Geometry: final body of the model. Coordinates: model frame, mm. Face numbers are marked on the shaded views. A direction names the side the tool comes from. Give positions to 0.01 mm unless a question says otherwise; leave off trailing zeros. Order: outer loops, then holes, each group sorted by start corner. A loop starts at its lowest first (then second) coordinate and runs counter-clockwise, first axis right, second up. Notation, with made-up numbers: M -17.5,-14 L 31.5,-14 A31 ccw 31.5,13 Z; hole C -32,89.5 d10. An arc over 180 degrees is marked long. One line per item, written item: value. Start each with the question number.
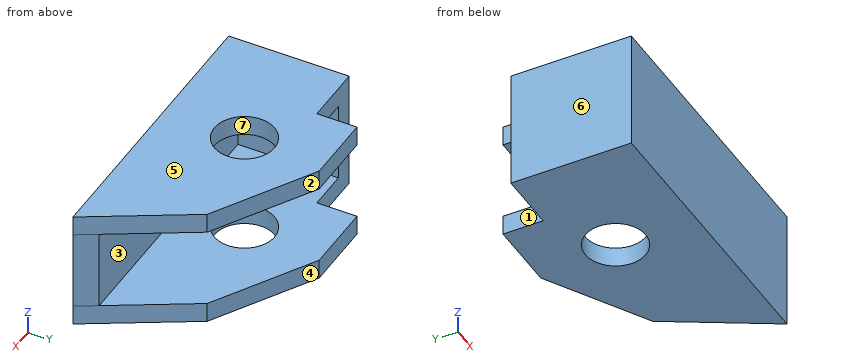
Autodesk Inventor part; units mm, degrees
ref_plane "YZ Plane" through (0, 0, 0) normal (1, 0, 0) x (0, 1, 0)
ref_plane "XZ Plane" through (0, 0, 0) normal (0, 1, 0) x (-1, 0, 0)
ref_plane "XY Plane" through (0, 0, 0) normal (0, 0, 1) x (1, 0, 0)
sketch "Sketch1" plane through (0, 0, 0) normal (0, 0, 1) x (1, 0, 0)
  line L0 (0, 0) -> (91.948, 0)
  line L1 (0, 0) -> (0, 38.1)
  line L2 (0, 38.1) -> (19.05, 38.1)
  line L3 (19.05, 38.1) -> (19.05, 50.8)
  line L4 (19.05, 50.8) -> (41.402, 50.8)
  line L5 (91.948, 0) -> (223.0777, 0) construction
  line L6 (41.402, 50.8) -> (73.2269, 32.4259)
  line L7 (91.948, 0) -> (73.2269, 32.4259)
  circle A0 centre (38.1, 25.4) radius 9.525
  dimension "d3" = 12.7
  dimension "d7" = 19.05
  dimension "d8" = 50.8
  dimension "d9" = 41.402
  dimension "d10" = 60
  dimension "d11" = 30
  dimension "d12" = 19.05
  dimension "d13" = 38.1
  dimension "d14" = 25.4
extrude "Extrusion1" add sketch "Sketch1" along normal blind 6.35
sketch "Sketch2" plane through (0, 0, 0) normal (0, 0, -1) x (-1, 0, 0)
  line L0 (-19.05, 38.1) -> (0, 38.1)
  line L1 (0, 0) -> (-6.35, 0)
  line L2 (-6.35, 0) -> (-6.35, 38.1)
  line L3 (-6.35, 38.1) -> (0, 38.1)
  line L4 (0, 38.1) -> (0, 0)
  dimension "d17" = 6.35
extrude "Extrusion2" add sketch "Sketch2" along normal blind 25.4
sketch "Sketch3" plane through (0, 0, 0) normal (0, 0, -1) x (-1, 0, 0)
  point P0 (0, 0)
sketch "Sketch4" plane through (0, 0, 0) normal (0, 0, -1) x (-1, 0, 0)
  line L0 (-6.35, 0) -> (-6.35, 6.35)
  line L1 (-6.35, 0) -> (-6.35, 38.1)
  line L2 (-6.35, 6.35) -> (-88.2818, 6.35)
  line L3 (-88.2818, 6.35) -> (-91.948, 0)
  line L4 (-91.948, 0) -> (-73.2269, 32.4259)
  line L5 (-91.948, 0) -> (-6.35, 0)
  line L6 (0, 0) -> (-91.948, 0)
  dimension "d21" = 6.35
extrude "Extrusion3" add sketch "Sketch4" along normal blind 25.4
sketch "Sketch5" plane through (0, 0, -25.4) normal (0, 0, -1) x (-1, 0, 0)
  point P0 (0, 0)
sketch "Sketch6" plane through (0, 0, -25.4) normal (0, 0, -1) x (-1, 0, 0)
  line L0 (0, 0) -> (0, 38.1)
  line L1 (0, 38.1) -> (-19.05, 38.1)
  line L2 (-19.05, 38.1) -> (-19.05, 50.8)
  line L3 (-19.05, 50.8) -> (-41.402, 50.8)
  line L4 (-41.402, 50.8) -> (-73.2269, 32.4259)
  line L5 (-73.2269, 32.4259) -> (-91.948, 0)
  line L6 (-91.948, 0) -> (0, 0)
  line L7 (0, 0) -> (-91.948, 0)
  circle A0 centre (-38.1, 25.4) radius 9.525
  dimension "d24" = 19.05
  dimension "d25" = 38.1
  dimension "d26" = 25.4
extrude "Extrusion4" add sketch "Sketch6" along normal blind 6.35
properties part number "2.4 Tutorial"
Q1. Section query B-B on z = 2. Return loops of the section in (x, y) (3 decimals).
Q2. Contact query for flat-ended pins moving along their axis: pin 1 (5 mm diameter, centred on y = 45, z = -27.5, fed in from -X); pin 2 (6 mm diameter, centred on y = 10, z = -21, fed in from +X); pin 3 (7.5 mm diameter, centred on x = 49, z = -17.5, fed in from +Y). Output: stop coordinate, or through.
Q3. Ray query, line 1 along Z through (x, y) = (23.5, 14); line 2 along Y through (x, z) = (38.1, -29.5) (3 decimals); line 3 along Y through (x, z) = (22.5, -2.5). Return the intervals inside material, ascending. Write a range as [from, to].
Q4. Section query A-A on x = 38.1. Return loops of the section in (y, z) (3 decimals).
Q5. Set-up query: the marked faces 1, 2 and 3. Return all of +Z, -Z, +X, -X, +Y, -Y with unobstructed straight access to the full face (end or side cutting, diameter ignored); none if empty.
Q6. Section query C-C on y = 40. Return loops of the section in (x, z), and give its area (3 significant figures).
Q7. Section query D-D on x = 8.5. Return loops of the section in (y, z), and give its area (3 significant figures).
Q8. Mould query, pull axis X, two halves, no side actions, for the marked faces 4, 5, 6 and 7. Classes: +X half, -X half, draft (parallel to the pull), parting line (faces both ways), or undercut.
Results below:
1. outline: M 0,0 L 91.948,0 L 73.227,32.426 L 41.402,50.8 L 19.05,50.8 L 19.05,38.1 L 0,38.1 Z; hole C 38.1,25.4 d19.05
2. pin 1: x = 19.05
2. pin 2: x = 6.35
2. pin 3: y = 6.35
3. line 1: [-31.75, -25.4], [0, 6.35]
3. line 2: [0, 15.875], [34.925, 50.8]
3. line 3: [0, 6.35]
4. outline: M 0,-31.75 L 15.875,-31.75 L 15.875,-25.4 L 6.35,-25.4 L 6.35,0 L 15.875,0 L 15.875,6.35 L 0,6.35 Z; M 34.925,-31.75 L 50.8,-31.75 L 50.8,-25.4 L 34.925,-25.4 Z; M 34.925,0 L 50.8,0 L 50.8,6.35 L 34.925,6.35 Z
5. face 1: +Z, -Z, -X, +Y
5. face 2: +Z, -Z, +X, +Y
5. face 3: +X, +Y
6. outline: M 19.05,-31.75 L 60.11,-31.75 L 60.11,-25.4 L 19.05,-25.4 Z; M 19.05,0 L 60.11,0 L 60.11,6.35 L 19.05,6.35 Z
6. area: 521 mm2
7. outline: M 0,-31.75 L 38.1,-31.75 L 38.1,-25.4 L 6.35,-25.4 L 6.35,0 L 38.1,0 L 38.1,6.35 L 0,6.35 Z
7. area: 645 mm2
8. face 4: +X half
8. face 5: draft
8. face 6: -X half
8. face 7: undercut
